Geometry: see drawing. Coordinates: mm, zero at the bounding-box minimum. A direction names the side the tool comes from. Coordinates: 2 decimals unless noted, no trailing zeros. Write each loop counter-clockwise with the first axis right and the second up, starting at its lowest first coordinate (ties: lowest second). Pieces come first, ordered by that corner, then holes. Notation, with made-up numbers: M -24.5,67 L 24.5,67 A17 ccw 24.5,82 Z; hole C -4,2 d4. An arc over 180 degrees is marked long. Answer as CSV lines item,"result". Start each with the question number.
1. Section B-B on z = 1.65. Return the cut outline in (x, y) (1 decimal).
2. Section D-D on z = 4.6. Return the cut outline in (x, y).
3. Section C-C on y = 1. Return the cut outline in (x, z), plus the area to 3 significant figures.
4. Line query: probe 1 along X at (y, z) = (13.25, 1.6) (1 decimal); probe 2 along X at (y, z) = (13.25, 3.25). Output: solid intervals per line, ascending. Write a range as [from, to].
5. Mould query, pull axis X, two halves, no side actions, for the marked faces 3, 4 and 5. Classes: pulls with the +X half, pulls with the -X half, needs draft (parallel to the pull), parting line crosses it, or undercut.
6. Section A-A on x = 13.5. Return the cut outline in (y, z).
7. Reachability of the marked faces 1 and 2 from +Z, -Z, +X, -X, +Y, -Y: full face, straight path, thin tool, end or side. Return the list, or none.
8. Contact query for flat-ended pins moving along their axis: pin 1 Ø3 at (x, z) = (22, 2) entering from +Y; pin 2 Ø2 at (x, y) = (5, 15.5) entering from +Z. Output: stop coordinate, or through.
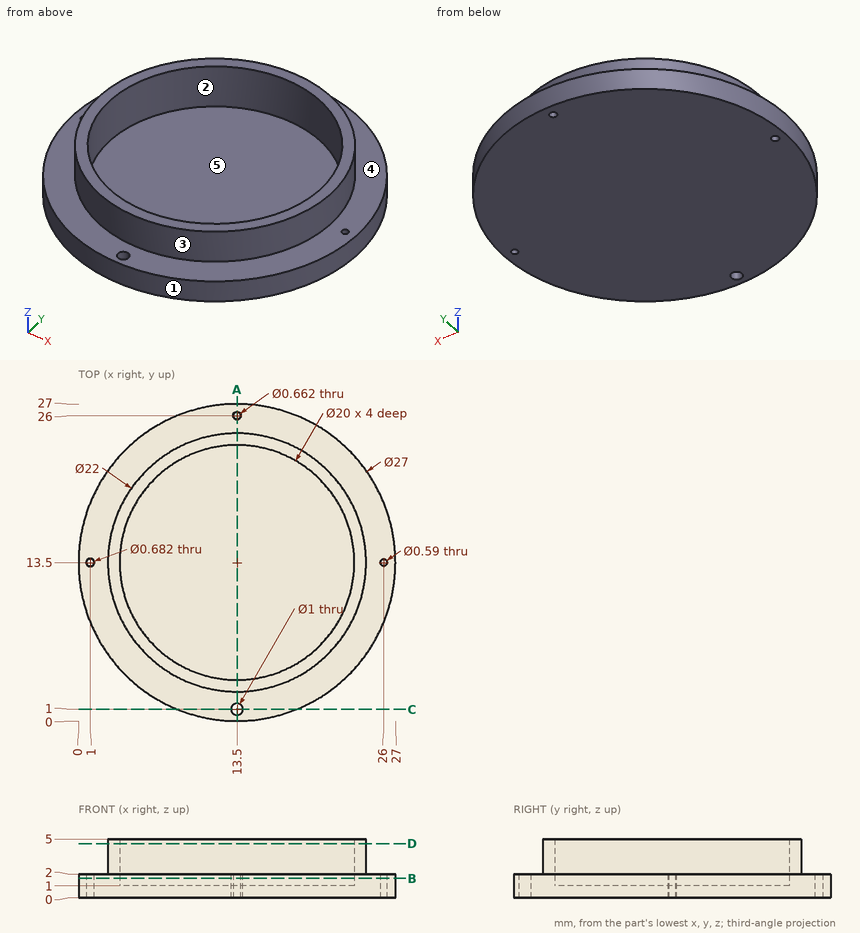
Values:
1,outline,"C 13.5,13.5 d27; hole C 1,13.5 d0.7; hole C 13.5,13.5 d20; hole C 13.5,1 d1; hole C 13.5,26 d0.7; hole C 26,13.5 d0.6"
2,outline,"C 13.5,13.5 d22; hole C 13.5,13.5 d20"
3,outline,"M 8.4,0 L 13,0 L 13,2 L 8.4,2 Z; M 14,0 L 18.6,0 L 18.6,2 L 14,2 Z"
3,area,"18.4 mm²"
4,probe 1,"[0, 0.8], [1.2, 3.5], [23.5, 25.8], [26.2, 27]"
4,probe 2,"[2.5, 3.5], [23.5, 24.5]"
5,face 3,"parting line crosses it"
5,face 4,"needs draft"
5,face 5,"undercut"
6,outline,"M 0,0 L 0.5,0 L 0.5,2 L 0,2 Z; M 1.5,0 L 25.67,0 L 25.67,2 L 24.5,2 L 24.5,5 L 23.5,5 L 23.5,1 L 3.5,1 L 3.5,5 L 2.5,5 L 2.5,2 L 1.5,2 Z; M 26.33,0 L 27,0 L 27,2 L 26.33,2 Z"
7,face 1,"+Z, -Z"
7,face 2,"+Z"
8,pin 1,"y = 25.04"
8,pin 2,"z = 1"
